from build123d import *

# Parameters (mm, degrees)
F1_DEPTH    = 30
F2_T1_DEPTH = 163.7053411471
F2_T3_DEPTH = 285.7735535498
F3_T1_DEPTH = 47.177253683
F4_W        = 30
F4_H        = 30
F5_DEPTH    = 400


# Not quite as in the source:
# - a fillet or chamfer that OpenCascade refuses, or shapes differently, is made with other operations: its cross-section is extruded or revolved along the edge and cut away or added


with BuildPart() as f1:
    # F0 (on Right) → F1 (new body)
    with BuildSketch(Plane.YZ):
        with BuildLine():
            Line((0.9376178496, 9.3718236312), (0, 0))
            Line((0, 0), (30, 0))
            Line((30, 0), (58.7747889852, 230.3266173388))
            ThreePointArc((58.7747889852, 230.3266173388), (62.2448009202, 267.4447024247), (63.4029619396, 304.7066385838))
            Line((63.4029619396, 304.7066385838), (63.4029619396, 375))
            Line((63.4029619396, 375), (59.769593104, 426.4305293125))
            Line((59.769593104, 426.4305293125), (16.7944896966, 824.9977231026))
            Line((16.7944896966, 824.9977231026), (16.6203579544, 825))
            Line((16.6203579544, 825), (-13.3796420456, 825))
            Line((-13.3796420456, 825), (29.9452786307, 423.188469929))
            ThreePointArc((29.9452786307, 423.188469929), (32.5379175275, 391.0741192729), (33.4029619396, 358.8668996991))
            Line((33.4029619396, 358.8668996991), (33.4029619396, 304.7066385838))
            ThreePointArc((33.4029619396, 304.7066385838), (32.3027089712, 269.3077992327), (29.0061976329, 234.0456184011))
            Line((29.0061976329, 234.0456184011), (0.9376178496, 9.3718236312))
        make_face()
    extrude(amount=F1_DEPTH)

    # F2: fillet of radius 1450 on 4 edges, made by hand

    # F2_s2 → F2_t1 (cut)
    with BuildSketch(Plane.YZ.offset(-66.8526705736)):
        with BuildLine():
            ThreePointArc((61.6540498994, 399.7559430432), (59.5240083024, 426.4086220464), (56.9028806071, 453.0174939664))
            Line((56.9028806071, 453.0174939664), (59.769593104, 426.4305293125))
            Line((59.769593104, 426.4305293125), (61.6540498994, 399.7559430432))
        make_face()
    extrude(amount=F2_T1_DEPTH, mode=Mode.SUBTRACT)

    # F2_s4 → F2_t3 (cut)
    with BuildSketch(Plane.YZ.offset(-127.8867767749)):
        with BuildLine():
            ThreePointArc((63.4029619396, 323.84528929), (62.5014570183, 374.968195708), (59.7980632353, 426.027533089))
            Line((59.7980632353, 426.027533089), (63.4029619396, 375))
            Line((63.4029619396, 375), (63.4029619396, 323.84528929))
        make_face()
    extrude(amount=F2_T3_DEPTH, mode=Mode.SUBTRACT)

    # F3: fillet of radius 300 on 4 edges, made by hand

    # F3_s2 → F3_t1 (cut)
    with BuildSketch(Plane.YZ.offset(-8.5886268415)):
        with BuildLine():
            ThreePointArc((60.3891403463, 416.3117677563), (60.6508457711, 412.8864247118), (60.8733107804, 409.4583094831))
            ThreePointArc((60.8733107804, 409.4583094831), (60.7708746607, 411.1729780567), (60.666407351, 412.8875240775))
            ThreePointArc((60.666407351, 412.8875240775), (60.5287879715, 414.5997280322), (60.3891403463, 416.3117677563))
        make_face()
    extrude(amount=F3_T1_DEPTH, mode=Mode.SUBTRACT)

    # F4 (on face) → F5 (join)
    with BuildSketch(Plane(origin=(0, 63.4029619396, 0), x_dir=(-1, 0, 0), z_dir=(0, 1, 0))):
        with Locations((-15, 308.84528929)):
            Rectangle(F4_W, F4_H)
    extrude(amount=F5_DEPTH)


solid = f1.part
Input: part model. Units: mm. Frame: model coordinates. A direction names the side the tool comes from. Give positions to 0.01 mm unless a question says otherwise; leave off trailing zeros. Write each loop counter-clockwise with the first axis right and the second up, starting at its lowest first coordinate (ties: lowest second). Pieces come first, ordered by that corner, then holes. Notation, with made-up numbers: M -36,7.25 L 15,7.25 A35 ccw 15,45.25 Z; hole C -20.75,41 d11. An arc over 180 degrees is marked long. Use one line per item in the form item = value.
1. Cut plane C-C on z = 600. Return loops of the section in (x, y), and give its area (3 significant figures).
Outcome:
outline = M 0,10.88 L 30,10.88 L 30,41.05 L 0,41.05 Z
area = 905 mm²
2. First-contact query: P1, Ø9, axis at x = 14.5, y = 231, coming from the +Z side; P2, Ø1.5, axis at x = 5, y = 237.5, coming from the -Z side; P3, Ø1, axis at x = 4.5, z = 183.5, coming from the +Y side. Flat tips, straight axial feed; report the tip coordinate or a pass-through.
Outcome:
P1 = 323.85
P2 = 293.85
P3 = 52.99
3. Cut plane B-B on y = 136.5. Return loops of the section in (x, z), and give its area (3 significant figures).
Outcome:
outline = M 0,293.85 L 30,293.85 L 30,323.85 L 0,323.85 Z
area = 900 mm²
4. Mould query, pull axis Z, two halves, no side actions, for faces 1 (the face through (15, 33.403, 332)), 2 (the face through (14.79, 44.186, 113.551)), 3 (the face through (14.79, 32.514, 391.525)), 4 (the face through (14.79, 58.787, 434.419)). Classes: released by +Z, released by -Z, zero draft, split by the parting line, or undercut.
Outcome:
face_1 = undercut
face_2 = released by -Z
face_3 = undercut
face_4 = released by +Z
5. Reachability of faces 5 (the face through (14.79, 15.17, 123.28)), 6 (the face through (15, 261, 323.845)), 7 (the face through (15, 15, 0)), 8 (the face through (15, 261, 293.845)) from +Z, -Z, +X, -X, +Y, -Y: full face, straight path, thin tool, end or side. Return the list, or none.
Outcome:
face_5 = +X, -X, -Y
face_6 = +Z, +X, -X, +Y
face_7 = -Z, +X, -X, +Y, -Y
face_8 = -Z, +X, -X, +Y
6. Ray query, L1, parallel to Z at x = 28, y = 366; L2, parallel to Y at x = 12, z = 387.5; L3, parallel to Y at x = 19.25, z = 678.5. Return the intervals inside material, ascending.
Outcome:
L1 = 293.85 to 323.85
L2 = 32.72 to 62.01
L3 = 2.42 to 32.59
7. Cut plane A-A on x = 10.5. Return loops of the section in (y, z).
Outcome:
outline = M -13.38,825 L 29.95,423.19 A600 cw 33.4,358.87 L 33.4,304.71 A570 cw 29.01,234.05 L 0.94,9.37 L 0,0 L 30,0 L 58.77,230.33 A600 ccw 63.4,304.71 L 63.4,293.85 L 463.4,293.85 L 463.4,323.85 L 63.4,323.85 A1450 ccw 60.87,409.46 A300 ccw 60.39,416.31 A1450 ccw 56.9,453.02 L 16.79,825 L 16.62,825 Z
